The listing builds one solid part. Answer for the finished solid, in the listing's coordinates (mm). A direction names the side the tool comes from. Give positions to 0.01 mm unless a question says otherwise; leave off trailing zeros. Order: outer loops, then holes, each group sorted by start corner. A loop starts at its lowest first (then second) coordinate and runs counter-clockwise, first axis right, second up. Notation, with made-up numbers: (64, 34) - (102, 34) arc R12 ccw to (102, 46) - close; hole circle Ø7 at (-0.5, 54). An arc over 180 degrees is marked (long way). Use a Markdown table: item, result. Add a question column.
1) For faces 4 (the face through (25.05, -23.57, -12.35)), 5 (the face through (-26, 13.8, -12)), 6 (the face through (18, 0, 0.5)), 7 (the face through (29.103, 12, -12)), 8 (the face through (0, -28, 0)), determine the directions among +Z, -Z, +X, -X, +Y, -Y from which every point of the face is accessible in a straight line to the end or side of a thin tool.
2) Find section B-B, the plane y = 12.5. Determine the outline of the cut face in (x, z), plus the area to 3 significant figures.
3) Find section A-A, the plane z = -2.75. Determine the outline of the cut face in (x, y).
4) Find section C-C, the plane x = -11.5. Determine the outline of the cut face in (y, z).
5) Flat-ended cylindrical pins translate along their axes: pin 1 (12 mm diameter, centred on x = -27, y = -12, fed in from -Z); pin 2 (10 mm diameter, centred on y = -19.5, z = -4.5, fed in from +X); pin 3 (6 mm diameter, centred on x = 25, z = -14.5, fed in from -Y); pin 4 (1.8 mm diameter, centred on x = -25, z = -8.5, fed in from -Y). Find the tip coordinate at first contact, or state that the pin passes through.
6) Straight lines are drawn through the part: line 1 (Y direction, x = 18, z = 1.2); line 2 (X direction, y = 24.5, z = -0.45); line 3 (Y direction, x = 23.5, z = -21.5). For each, find the intervals that lie inside material, in ascending order.
7) Find section D-D, the plane x = 17. Determine the outline of the cut face in (y, z).
8) The mould has two halves that part along X. Classify faces 1 (the face through (21.103, 12, -12)), 2 (the face through (-28.742, 12, -12)), 3 (the face through (23, -24.539, -12)): released by +X, released by -X, zero draft, split by the parting line, or undercut.
from build123d import *

# Parameters (mm, degrees)
ESQUISSE1_W                                    = 68
ESQUISSE1_H                                    = 56
BOSS_EXTRU_1_DEPTH                             = 1.5
ENL_V_MAT_EXTRU_1_REACH                        = 68.114
ESQUISSE2_R                                    = 2.5
CONG_1_R                                       = 3.5
FRAISAGE_POUR_VIS_T_TE_FRAIS_E_M31_D           = 3.4
FRAISAGE_POUR_VIS_T_TE_FRAIS_E_M31_DEPTH       = 21.67
FRAISAGE_POUR_VIS_T_TE_FRAIS_E_M31_CSINK_D     = 6.3
FRAISAGE_POUR_VIS_T_TE_FRAIS_E_M31_CSINK_ANGLE = 90
FRAISAGE_POUR_VIS_T_TE_FRAIS_E_M31_TIP         = 1.021463052
BOSS_EXTRU_2_DEPTH                             = 22
ENL_V_MAT_EXTRU_2_DEPTH                        = 2


with BuildPart() as part:
    # Esquisse1 → Boss.-Extru.1 (new, symmetric)
    with BuildSketch(Plane.XY):
        Rectangle(ESQUISSE1_W, ESQUISSE1_H)
    extrude(amount=BOSS_EXTRU_1_DEPTH, both=True)

    # Esquisse2 → Enlèv. mat.-Extru.1 (cut, up to next)
    with BuildSketch(Plane(origin=(-25.81698593, 0, 1.5), x_dir=(1, 0, 0), z_dir=(0, 0, 1)), mode=Mode.PRIVATE) as enl_v_mat_extru_1_sk1:
        with Locations((13.81698593, 0)):
            Circle(ESQUISSE2_R)
    enl_v_mat_extru_1_tool1 = extrude(enl_v_mat_extru_1_sk1.sketch, amount=-ENL_V_MAT_EXTRU_1_REACH, mode=Mode.PRIVATE) & part.part
    # Esquisse2 → Enlèv. mat.-Extru.1 (cut, up to next)
    with BuildSketch(Plane(origin=(-25.81698593, 0, 1.5), x_dir=(1, 0, 0), z_dir=(0, 0, 1)), mode=Mode.PRIVATE) as enl_v_mat_extru_1_sk2:
        with Locations((43.81698593, 6)):
            Circle(ESQUISSE2_R)
    enl_v_mat_extru_1_tool2 = extrude(enl_v_mat_extru_1_sk2.sketch, amount=-ENL_V_MAT_EXTRU_1_REACH, mode=Mode.PRIVATE) & part.part
    # Esquisse2 → Enlèv. mat.-Extru.1 (cut, up to next)
    with BuildSketch(Plane(origin=(-25.81698593, 0, 1.5), x_dir=(1, 0, 0), z_dir=(0, 0, 1)), mode=Mode.PRIVATE) as enl_v_mat_extru_1_sk3:
        with Locations((43.81698593, -6)):
            Circle(ESQUISSE2_R)
    enl_v_mat_extru_1_tool3 = extrude(enl_v_mat_extru_1_sk3.sketch, amount=-ENL_V_MAT_EXTRU_1_REACH, mode=Mode.PRIVATE) & part.part
    add(enl_v_mat_extru_1_tool1.solids().sort_by_distance((-12, 0, 1.5))[0], mode=Mode.SUBTRACT)
    add(enl_v_mat_extru_1_tool2.solids().sort_by_distance((18, 6, 1.5))[0], mode=Mode.SUBTRACT)
    add(enl_v_mat_extru_1_tool3.solids().sort_by_distance((18, -6, 1.5))[0], mode=Mode.SUBTRACT)

    # Congé1
    cong_1_edges = [part.edges().sort_by_distance(p)[0] for p in [
        (34, -28, 0),
        (-34, -28, 0),
        (-34, 28, 0),
        (34, 28, 0),
    ]]
    fillet(cong_1_edges, radius=CONG_1_R)

    # Fraisage pour vis à tête fraisée M31
    with Locations(Plane.XY.offset(1.5)):
        with Locations((-30.5, -24.5), (-30.5, 24.5), (30.5, 24.5), (30.5, -24.5)):
            CounterSinkHole(FRAISAGE_POUR_VIS_T_TE_FRAIS_E_M31_D / 2, FRAISAGE_POUR_VIS_T_TE_FRAIS_E_M31_CSINK_D / 2, depth=FRAISAGE_POUR_VIS_T_TE_FRAIS_E_M31_DEPTH, counter_sink_angle=FRAISAGE_POUR_VIS_T_TE_FRAIS_E_M31_CSINK_ANGLE)
            with Locations((0, 0, -(FRAISAGE_POUR_VIS_T_TE_FRAIS_E_M31_DEPTH + FRAISAGE_POUR_VIS_T_TE_FRAIS_E_M31_TIP / 2))):  # 118° drill point
                Cone(0, FRAISAGE_POUR_VIS_T_TE_FRAIS_E_M31_D / 2, FRAISAGE_POUR_VIS_T_TE_FRAIS_E_M31_TIP, mode=Mode.SUBTRACT)

    # Esquisse6 → Boss.-Extru.2 (add)
    with BuildSketch(Plane(origin=(0, 0, -1.5), x_dir=(-1, 0, 0), z_dir=(0, 0, -1))):
        Polygon((-21.103469563, -20.5), (-26, -20.5), (-26, -22.621320344), (-24.082132084, -24.539188259), (-21.103469563, -24.539188259), align=None)
        Polygon((22.741804985, 10.5), (27.5, 10.5), (28.741804985, 10.5), (28.741804985, 13.8), (22.741804985, 13.8), align=None)
        Polygon((-21.103469563, 10.5), (-26, 10.5), (-29.103469563, 10.5), (-29.103469563, 13.8), (-21.103469563, 13.8), align=None)
    extrude(amount=BOSS_EXTRU_2_DEPTH)

    # Esquisse7 → Enlèv. mat.-Extru.2 (cut)
    with BuildSketch(Plane(origin=(0, 0, -1.5), x_dir=(-1, 0, 0), z_dir=(0, 0, -1))):
        with BuildLine():
            Line((-23, -6), (-23, 6))
            ThreePointArc((-23, 6), (-18, 11), (-13, 6))
            Line((-13, 6), (-13, -6))
            ThreePointArc((-13, -6), (-18, -11), (-23, -6))
        make_face()
    extrude(amount=-ENL_V_MAT_EXTRU_2_DEPTH, mode=Mode.SUBTRACT)


solid = part.part
The answers:
| question | item | result |
|---|---|---|
| 1 | face 4 | -Z, +X, -Y |
| 1 | face 5 | -Z, +X, -X, +Y |
| 1 | face 6 | -Z |
| 1 | face 7 | -Z, +X, +Y, -Y |
| 1 | face 8 | +Z, -Z, +X, -X, -Y |
| 2 | outline | (-34, -1.5) - (-28.74, -1.5) - (-28.74, -23.5) - (-22.74, -23.5) - (-22.74, -1.5) - (21.1, -1.5) - (21.1, -23.5) - (29.1, -23.5) - (29.1, -1.5) - (34, -1.5) - (34, 1.5) - (-34, 1.5) - close |
| 2 | area | 512 mm2 |
| 3 | outline | (-28.74, 10.5) - (-22.74, 10.5) - (-22.74, 13.8) - (-28.74, 13.8) - close; (21.1, -24.54) - (24.08, -24.54) - (26, -22.62) - (26, -20.5) - (21.1, -20.5) - close; (21.1, 10.5) - (29.1, 10.5) - (29.1, 13.8) - (21.1, 13.8) - close |
| 4 | outline | (-28, -1.5) - (-2.45, -1.5) - (-2.45, 1.5) - (-28, 1.5) - close; (2.45, -1.5) - (28, -1.5) - (28, 1.5) - (2.45, 1.5) - close |
| 5 | pin 1 | z = -1.5 |
| 5 | pin 2 | x = 34 |
| 5 | pin 3 | y = -24.54 |
| 5 | pin 4 | y = 10.5 |
| 6 | line 1 | -28 to -8.5, -3.5 to 3.5, 8.5 to 28 |
| 6 | line 2 | -34 to -32.2, -28.8 to 28.8, 32.2 to 34 |
| 6 | line 3 | -24.54 to -20.5, 10.5 to 13.8 |
| 7 | outline | (-28, -1.5) - (-10.9, -1.5) - (-10.9, 0.5) - (-8.29, 0.5) - (-8.29, 1.5) - (-28, 1.5) - close; (-3.71, 0.5) - (3.71, 0.5) - (3.71, 1.5) - (-3.71, 1.5) - close; (8.29, 0.5) - (10.9, 0.5) - (10.9, -1.5) - (28, -1.5) - (28, 1.5) - (8.29, 1.5) - close |
| 8 | face 1 | undercut |
| 8 | face 2 | released by -X |
| 8 | face 3 | zero draft |
